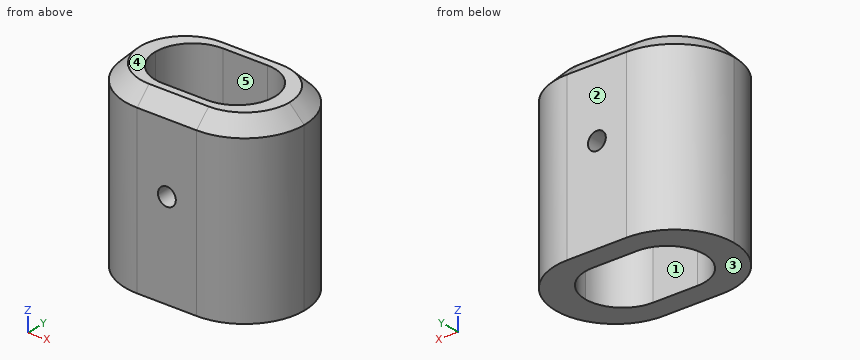
```python
from build123d import *

# Parameters (mm, degrees)
F1_DEPTH = 60
F2_SIZE  = 5
F3_R     = 3
F4_DEPTH = 40.001


with BuildPart() as f1:
    # F0 (on Top) → F1 (new body)
    with BuildSketch(Plane.XY):
        with BuildLine():
            ThreePointArc((30, 0), (24.1421356237, 14.1421356237), (10, 20))
            Line((10, 20), (-10, 20))
            ThreePointArc((-10, 20), (-24.1421356237, 14.1421356237), (-30, 0))
            ThreePointArc((-30, 0), (-24.1421356237, -14.1421356237), (-10, -20))
            Line((-10, -20), (10, -20))
            ThreePointArc((10, -20), (24.1421356237, -14.1421356237), (30, 0))
        make_face()
        with BuildLine():
            Line((-7.5, 12.5), (7.5, 12.5))
            ThreePointArc((7.5, 12.5), (16.3388347648, 8.8388347648), (20, 0))
            ThreePointArc((20, 0), (16.3388347648, -8.8388347648), (7.5, -12.5))
            Line((7.5, -12.5), (-7.5, -12.5))
            ThreePointArc((-7.5, -12.5), (-16.3388347648, -8.8388347648), (-20, 0))
            ThreePointArc((-20, 0), (-16.3388347648, 8.8388347648), (-7.5, 12.5))
        make_face(mode=Mode.SUBTRACT)
    extrude(amount=F1_DEPTH)

    # F2
    f2_edges = [f1.edges().sort_by_distance(p)[0] for p in [
        (30, 0, 60),
        (0, 20, 60),
        (-30, 0, 60),
        (0, -20, 60),
    ]]
    chamfer(f2_edges, length=F2_SIZE)

    # F3 (on face) → F4 (cut, through all)
    with BuildSketch(Plane.XZ.offset(20)):
        with Locations((0, 32)):
            Circle(F3_R)
    extrude(amount=-F4_DEPTH, mode=Mode.SUBTRACT)


solid = f1.part
```
The listing builds one solid part. Answer for the finished solid, in the listing's coordinates (mm). Face numbers are marked on the shaded views. A direction names the side the tool comes from. Round coordinates to 2 decimals unless told otherwise and drop trailing zeros. Loops run counter-clockwise (first coordinate to the right, second up) from the corner with the lowest first, then second, coordinate; pieces in that order, holes last.
1) A cutting plane is placed at B-B on x = 0. Determine the outline of the cut face in (y, z), plus the area to 3 significant figures.
Outcome:
outline: (-20, 0) - (-12.5, 0) - (-12.5, 29) - (-20, 29) - close; (-20, 35) - (-12.5, 35) - (-12.5, 60) - (-15, 60) - (-20, 55) - close; (12.5, 0) - (20, 0) - (20, 29) - (12.5, 29) - close; (12.5, 35) - (20, 35) - (20, 55) - (15, 60) - (12.5, 60) - close
area: 785 mm2
2) A cutting plane is placed at C-C on z = 32. Determine the outline of the cut face in (x, y).
Outcome:
outline: (-10, -20) - (-3, -20) - (-3, -12.5) - (-7.5, -12.5) arc R12.5 cw to (-7.5, 12.5) - (-3, 12.5) - (-3, 20) - (-10, 20) arc R20 ccw to start; (3, -20) - (10, -20) arc R20 ccw to (10, 20) - (3, 20) - (3, 12.5) - (7.5, 12.5) arc R12.5 cw to (7.5, -12.5) - (3, -12.5) - close
3) For a pull along Y with two mould halves and no side action, classify the marked faces 1, 2 and 3 as released by +Y, released by -Y, zero draft, split by the parting line, or undercut.
Outcome:
face 1: undercut
face 2: released by +Y
face 3: zero draft
4) Consider line 1 (Y direction, x = 3.5, z = 14); line 2 (Z direction, x = 0, y = -16); line 3 (Y direction, x = 10, z = 8). Determine where each line is inside the solid, lowest interval first.
Outcome:
line 1: y = -20 to -12.5, 12.5 to 20
line 2: z = 0 to 29, 35 to 59
line 3: y = -20 to -12.25, 12.25 to 20
5) A cutting plane is placed at A-A on z = 17. Determine the outline of the cut face in (x, y).
Outcome:
outline: (-10, -20) - (10, -20) arc R20 ccw to (10, 20) - (-10, 20) arc R20 ccw to start; hole (-7.5, -12.5) - (7.5, -12.5) arc R12.5 ccw to (7.5, 12.5) - (-7.5, 12.5) arc R12.5 ccw to start
6) Given P1, Ø3, axis at x = 20.5, z = 14, coming from the +Y side; P2, Ø1.5, axis at y = 9, z = 12.5, coming from the -X side; P3, Ø1, axis at x = 14, z = 34.5, coming from the +Y side; P4, Ø5.5, axis at x = 0, z = 32, coming from the -Y side, each flat-ended and moving along its own axis, determine where each tip first touches the part or whether it passes through.
Outcome:
P1: stops at y = 17.86
P2: stops at x = -28.22
P3: stops at y = 19.69
P4: passes through
7) For the marked faces 4 and 5, determine the directions among +Z, -Z, +X, -X, +Y, -Y from which every point of the face is accessible in a straight line to the end or side of a thin tool.
Outcome:
face 4: +Z, +X, -X, +Y, -Y
face 5: +Z, -Z
